Verification items for the finished model (mm, model axes). Coordinates: 2 decimals unless noted, no trailing zeros. Write each loop counter-clockwise with the first axis right and the second up, starting at its lowest first coordinate (ties: lowest second). Pieces come first, ordered by that corner, then holes. Notation, with made-up numbers: (-32, 54) -> (-13, 54) arc R23 ccw to (-13, 93) -> close; hole circle Ø6 at (5.25, -24). An arc over 180 degrees is marked (long way). Write item = value, one per line. Start each with the question number.
(1) Material ranges on probe 1 along Z at (x, y) = (0.3, 0); probe 2 along Y at (x, z) = (0.2, 10); probe 3 along Z at (x, y) = (1.35, 0.7), recorded low to high. Write a range as [from, to].
(2) Gauge pin test, flat end, axial feed: pin 1 Ø1.4 at (y, z) = (0, 71) entering from +X. Record the tip position at first contact, or that the pin passes through.
(3) Section check A-A (z = 34.5). Record the cut outline in (x, y).
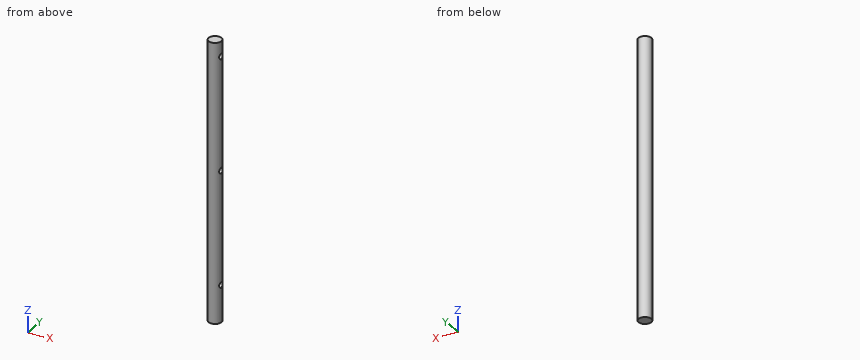
Autodesk Inventor part; units mm, degrees
ref_plane "Arbeitsebene2" through (1.75, 0, 0) normal (1, 0, 0) x (0, 1, 0)
ref_plane "XZ Plane" through (0, 0, 0) normal (0, 1, 0) x (-1, 0, 0)
ref_plane "XY Plane" through (0, 0, 0) normal (0, 0, 1) x (1, 0, 0)
sketch "Skizze1" plane through (0, 0, 0) normal (0, 0, 1) x (1, 0, 0)
  circle A0 centre (0, 0) radius 1.75
  dimension "d0" = 3.5
extrude "Extrusion1" add sketch "Skizze1" along normal blind 75
ref_plane "Arbeitsebene2" through (1.75, 0, 0) normal (1, 0, 0) x (0, 1, 0)
sketch "Skizze8" plane through (1.75, 0, 0) normal (1, 0, 0) x (0, 1, 0)
  line L0 (0, 0) -> (0, 10) construction
  line L1 (0, 10) -> (0, 40.5) construction
  line L2 (0, 40.5) -> (0, 71) construction
  dimension "d14" = 10
  dimension "d15" = 30.5
  dimension "d16" = 30.5
hole "Bohrung2" at (1.75, 0, 10) at (1.75, 0, 40.5) at (1.75, 0, 71) at (1.75, 0, 10) at (1.75, 0, 40.5) at (1.75, 0, 71) direction (-1, 0, 0) diameter 1.6 depth 2 tip angle 118
properties part number "cu_stange"
Response:
q1.probe_1 = [0, 9.2], [10.8, 39.7], [41.3, 70.2], [71.8, 75]
q1.probe_2 = [-1.74, -0.8], [0.8, 1.74]
q1.probe_3 = [0, 9.61], [10.39, 40.11], [40.89, 70.61], [71.39, 75]
q2.pin_1 = -0.31
q3.outline = circle Ø3.5 at (0, 0)
